from build123d import *

# Parameters (mm, degrees)
SKETCH_1_R          = 11.5
EXTRUDE_1_DEPTH     = 2.3
SKETCH_2_R          = 11.5
EXTRUDE_2_DEPTH     = 0.7
SKETCH_3_R          = 5
CUT_EXTRUDE_1_DEPTH = 10


with BuildPart() as part:
    # 草图1 → 凸台-拉伸1 (new body)
    with BuildSketch(Plane.XY):
        Circle(SKETCH_1_R)
        Polygon((8, -3.175426481), (10.75, -1.58771324), (10.75, 1.58771324), (8, 3.175426481), (5.25, 1.58771324), (5.25, -1.58771324), align=None, mode=Mode.SUBTRACT)
        Polygon((3.175426481, 8), (1.58771324, 10.75), (-1.58771324, 10.75), (-3.175426481, 8), (-1.58771324, 5.25), (1.58771324, 5.25), align=None, mode=Mode.SUBTRACT)
        Polygon((-3.175426481, -8), (-1.58771324, -10.75), (1.58771324, -10.75), (3.175426481, -8), (1.58771324, -5.25), (-1.58771324, -5.25), align=None, mode=Mode.SUBTRACT)
        Polygon((-8, 3.175426481), (-10.75, 1.58771324), (-10.75, -1.58771324), (-8, -3.175426481), (-5.25, -1.58771324), (-5.25, 1.58771324), align=None, mode=Mode.SUBTRACT)
    extrude(amount=EXTRUDE_1_DEPTH)

    # 草图2 → 凸台-拉伸2 (add)
    with BuildSketch(Plane.XY.offset(2.3)):
        Circle(SKETCH_2_R)
    extrude(amount=EXTRUDE_2_DEPTH)

    # 草图3 → 切除-拉伸1 (cut)
    with BuildSketch(Plane.XY.offset(3)):
        Circle(SKETCH_3_R)
    extrude(amount=-CUT_EXTRUDE_1_DEPTH, mode=Mode.SUBTRACT)


solid = part.part
Can you work these out from the model? Positions are in its coordinate system, mm. A direction names the side the tool comes from. Round coordinates to 2 decimals unless told otherwise and drop trailing zeros. Write each loop counter-clockwise with the first axis right and the second up, starting at its lowest first coordinate (ties: lowest second). Pieces come first, ordered by that corner, then holes. Notation, with made-up numbers: (85, 35) -> (121, 35) arc R18 ccw to (121, 54) -> close; hole circle Ø10 at (47.25, 59.25). An arc over 180 degrees is marked (long way). Use one line per item in the form item = value. Start each with the question number.
Q1. Imagine slicing it at C-C (z = 1.6). Please give me the cut outline in (x, y).
Q2. Which directions (+Z, -Z, +X, -X, +Y, -Y) give clear straight access to the entire face, cutting with the end or side of a thin tool? Please do faces 4 (the face through (-5.25, 0, 1)), 5 (the face through (-1.08, -4.88, 1.52)).
Q3. If I drill on probe 1 along Y at (x, z) = (0, 1.3); probe 2 along X at (y, z) = (3, 1.45); probe 3 along Y at (x, z) = (-0.75, 1.2), over which ranges is the centre line in solid material (lowest first)? Write a range as [from, to].
Q4. I'm going to push flat-ended pins straight in: P1, Ø1.5, axis at x = 5, z = 0.5, coming from the -Y side; P2, Ø1.6, axis at x = -0.5, y = -7, coming from the -Z side. Where does each tip first touch, or does it pass through?
Q5. Imagine slicing it at A-A (x = 0). Please give me the cut outline in (y, z), then the cut area to 3 significant figures.
Q6. Imagine slicing it at D-D (y = 4). Please give me the cut outline in (x, z), then the cut area to 3 significant figures.
Q7. We'd pull the mould along X, two halves only. Please class faces 1 (the face through (-1.5, 11.4, 1.5)), 2 (the face through (-6.64, -2.39, 1.13)), 3 (the face through (5, -2, 3)): +X half, -X half, draft (parallel to the pull), parting line (faces both ways), or undercut.
Worked out:
q1.outline = circle Ø23 at (0, 0); hole (-10.75, -1.59) -> (-8, -3.18) -> (-5.25, -1.59) -> (-5.25, 1.59) -> (-8, 3.18) -> (-10.75, 1.59) -> close; hole circle Ø10 at (0, 0); hole (-3.18, -8) -> (-1.59, -10.75) -> (1.59, -10.75) -> (3.18, -8) -> (1.59, -5.25) -> (-1.59, -5.25) -> close; hole (-3.18, 8) -> (-1.59, 5.25) -> (1.59, 5.25) -> (3.18, 8) -> (1.59, 10.75) -> (-1.59, 10.75) -> close; hole (5.25, -1.59) -> (8, -3.18) -> (10.75, -1.59) -> (10.75, 1.59) -> (8, 3.18) -> (5.25, 1.59) -> close
q2.face_4 = -Z
q2.face_5 = +Z, -Z
q3.probe_1 = [-11.5, -10.75], [-5.25, -5], [5, 5.25], [10.75, 11.5]
q3.probe_2 = [-11.1, -8.3], [-7.7, -4], [4, 7.7], [8.3, 11.1]
q3.probe_3 = [-11.48, -10.75], [-5.25, -4.94], [4.94, 5.25], [10.75, 11.48]
q4.P1 = -10.69
q4.P2 = 2.3
q5.outline = (-11.5, 0) -> (-10.75, 0) -> (-10.75, 2.3) -> (-5.25, 2.3) -> (-5.25, 0) -> (-5, 0) -> (-5, 3) -> (-11.5, 3) -> close; (5, 0) -> (5.25, 0) -> (5.25, 2.3) -> (10.75, 2.3) -> (10.75, 0) -> (11.5, 0) -> (11.5, 3) -> (5, 3) -> close
q5.area = 13.7 mm^2
q6.outline = (-10.78, 0) -> (-3, 0) -> (-3, 3) -> (-10.78, 3) -> close; (3, 0) -> (10.78, 0) -> (10.78, 3) -> (3, 3) -> close
q6.area = 46.7 mm^2
q7.face_1 = parting line
q7.face_2 = undercut
q7.face_3 = draft
